Input: part model. Units: mm. Frame: model coordinates. Face numbers are marked on the shaded views. A direction names the side the tool comes from. Coordinates: 2 decimals unless noted, no trailing zeros. Write each loop counter-clockwise with the first axis right and the second up, starting at its lowest first coordinate (ties: lowest second). Pieces come first, ordered by that corner, then holes. Notation, with made-up numbers: M -3,16.5 L 28,16.5 A36 cw 28,54.5 Z; hole C -24.5,4.25 d2. An arc over 180 degrees is marked long. Use CSV: the item, a comma, the result in double quotes.
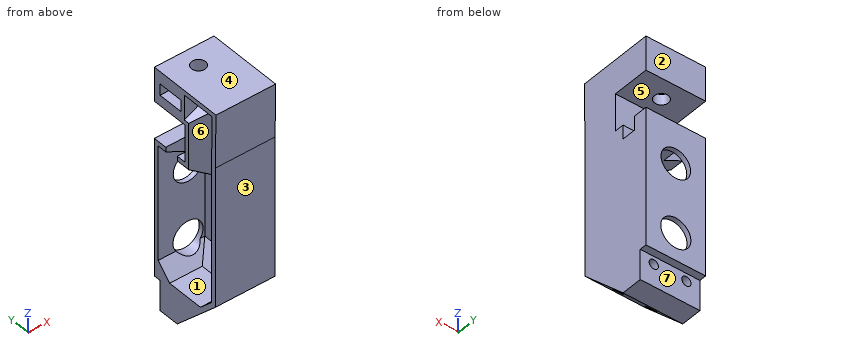
```python
from build123d import *

# Parameters (mm, degrees)
F0_W      = 5.55
F0_H      = 2.45
F1_DEPTH  = 6.4
F3_DEPTH  = 9.3
F2_R      = 1.5
F4_DEPTH  = 11.8
F5_DEPTH  = 3
F6_SIZE   = 10
F9_DEPTH  = 10
F10_R     = 1
F11_DEPTH = 16.7
F13_SIZE  = 3
F12_R     = 3.1718540483
F12_R_2   = 3.2332055741
F14_DEPTH = 11.3
F15_SIZE2 = 9.99999
F15_SIZE  = 4.99999


# Not quite as in the source:
# - a fillet or chamfer is up to 0.001 mm smaller than in the source, because OpenCascade refuses the exact size
# - a feature names something its author has since deleted; it is built from what else it names


with BuildPart() as f1:
    # F0 (on Right) → F1 (new body, symmetric)
    with BuildSketch(Plane.YZ):
        Polygon((-8, -3.8421934836), (-8, 0), (-16, 0), (-16, -40), (-1.5, -40), (-1.5, -33.5), (0, -33.5), (0, -3.8421934836), (-3, -3.8421934836), (-3, -6.8521934836), (-6.01, -6.8521934836), (-6.01, -3.8421934836), align=None)
        Polygon((-8, 4.1578065164), (0, 4.1578065164), (0, 8.6438981816), (0, 11.5000782534), (-16.1481745615, 11.5000782534), (-16, 0), (-8, 0), align=None)
        with Locations((-4.2636177904, 7.6219322528)):
            Rectangle(F0_W, F0_H, mode=Mode.SUBTRACT)
        with Locations((-4.2636177904, 7.6219322528)):
            Rectangle(F0_W, F0_H)
    extrude(amount=F1_DEPTH, both=True)

    # F0 (on Right) → F3 (cut)
    with BuildSketch(Plane.YZ):
        with Locations((-4.2636177904, 7.6219322528)):
            Rectangle(F0_W, F0_H)
    extrude(amount=-F3_DEPTH, mode=Mode.SUBTRACT)

    # F2 (on face) → F4 (cut)
    with BuildSketch(Plane.XY.offset(11.5000782534)):
        with Locations((-0.4, -4.2524)):
            Circle(F2_R)
    extrude(amount=-F4_DEPTH, mode=Mode.SUBTRACT)

    # F0 (on Right) → F5 (cut)
    with BuildSketch(Plane.YZ):
        with Locations((-4.2636177904, 7.6219322528)):
            Rectangle(F0_W, F0_H)
    extrude(amount=F5_DEPTH, mode=Mode.SUBTRACT)

    # F6
    f6_edges = [f1.edges().sort_by_distance(p)[0] for p in [
        (0, -16, -40),
    ]]
    chamfer(f6_edges, length=F6_SIZE)

    # F7 (on face) → F9 (cut)
    with BuildSketch(Plane(origin=(-6.4, 0, 0), x_dir=(0, -1, 0), z_dir=(-1, 0, 0))):
        Polygon((3, -6.8521934836), (3, -4.8421934836), (1, -4.8421934836), (1, -14.3586024642), (1, -21.1353842169), (1, -32.5), (2.5, -32.5), (12.0857864376, -32.5), (15, -29.5857864376), (15, 0.006442061), (15.135206901, 10.5000782534), (7.8539028764, 10.5000782534), (7.8539028764, 5.1578065164), (9, 5.1578065164), (9, -4.8421934836), (6.01, -4.8421934836), (6.01, -6.8521934836), align=None)
    extrude(amount=-F9_DEPTH, mode=Mode.SUBTRACT)

    # F10 (on face) → F11 (cut)
    with BuildSketch(Plane(origin=(0, -1.5, 0), x_dir=(-1, 0, 0), z_dir=(0, 1, 0))):
        with Locations((-3.5, -35.2)):
            Circle(F10_R)
        with Locations((3.5, -35.2)):
            Circle(F10_R)
    extrude(amount=-F11_DEPTH, mode=Mode.SUBTRACT)

    # F13
    f13_edges = [f1.edges().sort_by_distance(p)[0] for p in [
        (3.6, -6.542893, -32.5),
        (-1.4, -1, -32.5),
    ]]
    chamfer(f13_edges, length=F13_SIZE)

    # F12 (on face) → F14 (cut)
    with BuildSketch(Plane(origin=(0, 0, 0), x_dir=(-1, 0, 0), z_dir=(0, 1, 0))):
        with Locations((0, -12.6159423962)):
            Circle(F12_R)
        with Locations((0, -27.5774579495)):
            Circle(F12_R_2)
    extrude(amount=-F14_DEPTH, mode=Mode.SUBTRACT)

    # F15 (size 5 and 10 in the source; OpenCascade refuses exactly that, so slightly less here)
    f15_edges = [f1.edges().sort_by_distance(p)[0] for p in [
        (3.6, -7.505, -4.842193),
        (3.6, -9, 0.157807),
        (3.6, -8.426951, 5.157807),
    ]]
    f15_side = f1.faces().sort_by_distance((3.6, -8.906235, -12.735974))[0]
    chamfer(f15_edges, length=F15_SIZE, length2=F15_SIZE2, reference=f15_side)


solid = f1.part
```
1. Contact query for a flat-ended pin moving along its axis: pin 1 Ø7 at (x, z) = (1.5, -38) entering from +Y. Output: stop coordinate, or through.
Resolved:
pin 1,"stops at y = -1.5"
2. Section A-A (z = -35.2). Return loops of the section in (x, y), then the cut area to 3 significant figures.
Resolved:
outline,"M -6.4,-10.8 L -4.5,-10.8 L -4.5,-1.5 L -6.4,-1.5 Z; M -2.5,-10.8 L 2.5,-10.8 L 2.5,-1.5 L -2.5,-1.5 Z; M 4.5,-10.8 L 6.4,-10.8 L 6.4,-1.5 L 4.5,-1.5 Z"
area,"81.8 mm^2"
3. Access query for the marked faces 5, 6 and 7. Directions: +Z, -Z, +X, -X, +Y, -Y. A direction counts if a zero-diameter tool reaches every point of the face in a straight line with its end or side. Return the directions, or none.
Resolved:
face 5,"+X, -X, +Y"
face 6,"-X"
face 7,"-Z, +X, -X, +Y"
4. Section C-C (y = -9.5). Return loops of the section in (x, z).
Resolved:
outline,"M -6.4,-36.5 L 6.4,-36.5 L 6.4,11.5 L -6.4,11.5 L -6.4,10.5 L 3.6,10.5 L 3.6,10.16 L -5.4,5.66 L -5.4,-5.34 L 3.6,-9.84 L 3.6,-29.5 L 0.6,-32.5 L -6.4,-32.5 Z; hole C -3.5,-35.2 d2; hole C 3.5,-35.2 d2"
5. Material intervals for line 1 (Z direction, x = 0, y = -0.45); line 2 (X direction, y = -4.5, z = -35.2); line 3 (Z direction, x = 3.75, y = -5.75), sorted ascending. Write a range as [from, to].
Resolved:
line 1,"z = [-33.5, -30.81], [-24.34, -15.79], [-9.44, -3.84], [4.16, 11.5]"
line 2,"x = [-6.4, -4.5], [-2.5, 2.5], [4.5, 6.4]"
line 3,"z = [-40, -36.17], [-34.23, -6.85], [4.16, 11.5]"
6. Mould query, pull axis Y, two halves, no side actions, for the marked faces 1, 2, 3 and 4. Classes: pulls with the +Y half, pulls with the -Y half, needs draft (parallel to the pull), parting line crosses it, or undercut.
Resolved:
face 1,"undercut"
face 2,"pulls with the +Y half"
face 3,"pulls with the -Y half"
face 4,"needs draft"
